Design review of the part shown in the three views and the two pictorial views. Dimensions are in mm from the part's minimum x, y and z. Round coordinates to 2 decimals unless told otherwise and drop trailing zeros. Loops run counter-clockwise (first coordinate to the right, second up) from the corner with the lowest first, then second, coordinate; pieces in that order, holes last. Notation, with made-up numbers: M 51.5,67.25 L 68.5,67.25 A25 ccw 68.5,90.25 Z; hole C 37,-14 d4. An arc over 180 degrees is marked long. Return JSON: item names as keys, results as strings. Group by question number.
Q1. Consider section A-A (y = 11). State the section outline as (x, z) points, and give its area (3 significant figures).
Q2. To check wall thickness, follow line 1 along X through (y, z) = (16.75, 12); line 2 along X through (y, z) = (14.5, 8.5); line 3 along Y through (x, z) = (16.25, 13). State the ranges of each line that lie inside material, in increasing order.
Q3. Consider section B-B (z = 9.5). State the section outline as (x, y) points.
Q4. Consider section C-C (z = 2.25). State the section outline as (x, y) points, and give its area (3 significant figures).
Q5. Draft analysis for pull direction X (two halves, no side actions). For the marked faces 1, 2 and 3, state which applies: pulls with the +X half, pulls with the -X half, needs draft (parallel to the pull), parting line crosses it, or undercut.
Q6. Clearance check with flat-ended pins moving along their axes: pin 1 Ø1.5 at (x, z) = (15, 7.5) entering from +Y; pin 2 Ø8 at (y, z) = (6, 5.5) entering from -X; pin 3 Ø2 at (x, y) = (18.5, 3.5) entering from +Z; pin 4 Ø8 at (x, y) = (11, 11) entering from +Z. State where each tip first meets the part, or that it passes through.
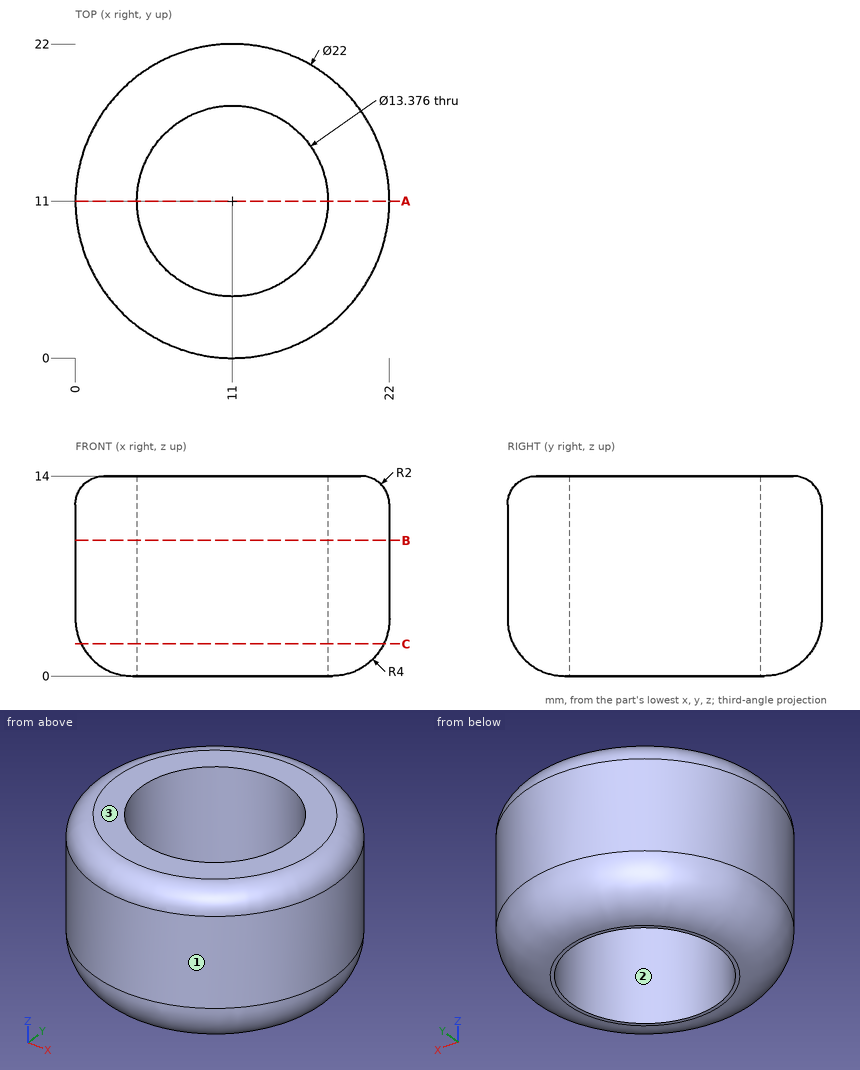
Values:
{
 "1": {"outline": "M 0,4 A4 ccw 4,0 L 4.31,0 L 4.31,14 L 2,14 A2 ccw 0,12 Z; M 17.69,0 L 18,0 A4 ccw 22,4 L 22,12 A2 ccw 20,14 L 17.69,14 Z", "area": "112 mm2"},
 "2": {"line 1": "x = 1.62 to 7.58, 14.42 to 20.38", "line 2": "x = 0.57 to 5.3, 16.7 to 21.43", "line 3": "y = 1.64 to 6.86, 15.14 to 20.36"},
 "3": {"outline": "C 11,11 d22; hole C 11,11 d13.38"},
 "4": {"outline": "C 11,11 d21.19; hole C 11,11 d13.38", "area": "212 mm2"},
 "5": {"face 1": "parting line crosses it", "face 2": "undercut", "face 3": "needs draft"},
 "6": {"pin 1": "stops at y = 21.51", "pin 2": "stops at x = 0.05", "pin 3": "stops at z = 13.91", "pin 4": "passes through"}
}
